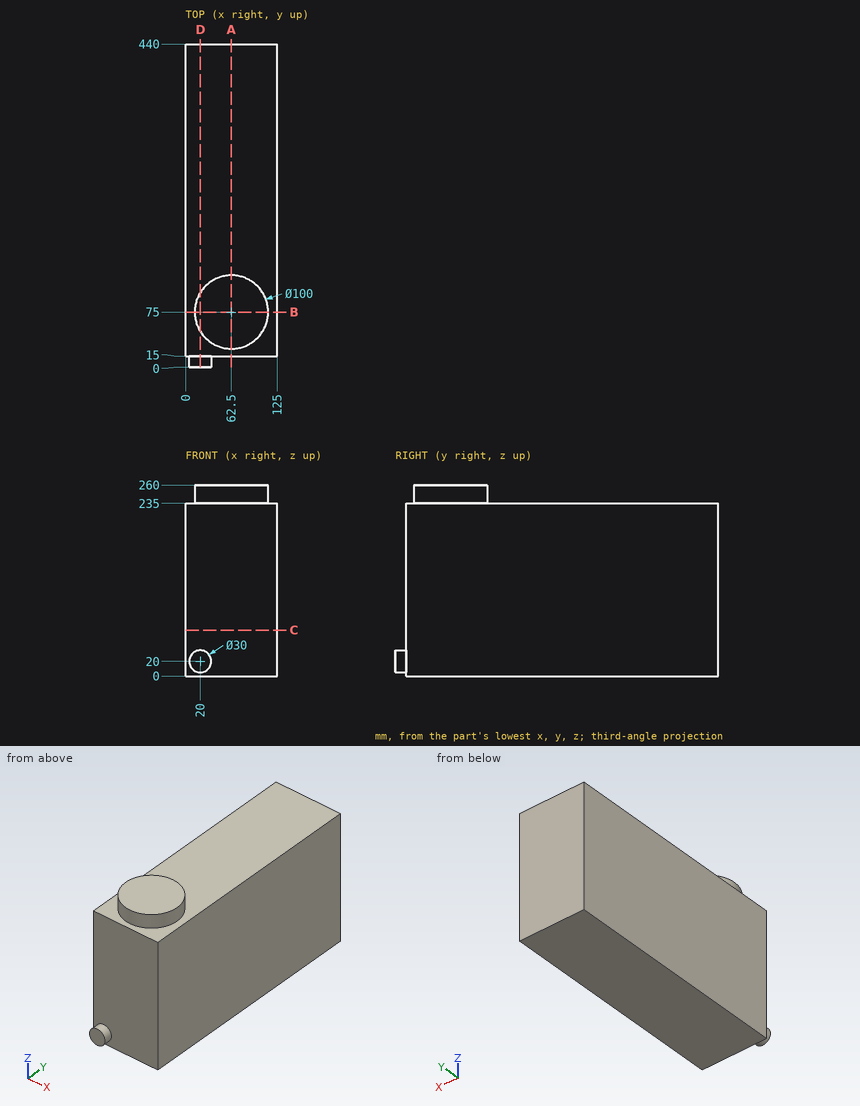
Here's the drawing with two shaded views (mm, measured from the low corner). I have some questions. Give positions to 0.01 mm unless a question says otherwise; leave off trailing zeros. Write each loop counter-clockwise with the first axis right and the second up, starting at its lowest first coordinate (ties: lowest second). Pieces come first, ordered by that corner, then holes. Notation, with made-up numbers: (69.5, -7) -> (127.5, -7) arc R29 ccw to (127.5, 23) -> close; hole circle Ø7 at (29.25, 14). An arc over 180 degrees is marked (long way). One line per item, written item: value.
Q1. For P1, Ø6, axis at x = 106, z = 43.5, coming from the -Y side, with a flat end and sliding along its axis, tell me the tip position at first contact or that it passes through.
Results found:
P1: stops at y = 15
Q2. Imagine slicing it at D-D on x = 20. Please give me the cut outline in (y, z).
Results found:
outline: (0, 5) -> (15, 5) -> (15, 0) -> (440, 0) -> (440, 235) -> (101.34, 235) -> (101.34, 260) -> (48.66, 260) -> (48.66, 235) -> (15, 235) -> (15, 35) -> (0, 35) -> close
Q3. Imagine slicing it at C-C on z = 62.5. Please give me the cut outline in (x, y).
Results found:
outline: (0, 15) -> (125, 15) -> (125, 440) -> (0, 440) -> close
Q4. Imagine slicing it at B-B on y = 75. Please give me the cut outline in (x, z), and give its area (3 significant figures).
Results found:
outline: (0, 0) -> (125, 0) -> (125, 235) -> (112.5, 235) -> (112.5, 260) -> (12.5, 260) -> (12.5, 235) -> (0, 235) -> close
area: 31,900 mm^2
Q5. Imagine slicing it at A-A on x = 62.5. Please give me the cut outline in (y, z), and give its area (3 significant figures).
Results found:
outline: (15, 0) -> (440, 0) -> (440, 235) -> (125, 235) -> (125, 260) -> (25, 260) -> (25, 235) -> (15, 235) -> close
area: 102,000 mm^2
Q6. Please list where these lines run through material, in increasing order: line 1 (Z direction, x = 40, y = 200); line 2 (Y direction, x = 97, z = 96). Write a range as [from, to].
Results found:
line 1: z = [0, 235]
line 2: y = [15, 440]
